Could you check a few things on this model? Use its own coordinates, in mm. Round coordinates to 2 decimals unless told otherwise and drop trailing zeros. Write each loop counter-clockwise with the first axis right and the second up, starting at its lowest first coordinate (ties: lowest second). Pieces come first, ordered by that corner, then holes. Notation, with made-up numbers: (-6.75, -28) -> (-2.75, -28) arc R7 ccw to (-2.75, -16) -> close; hole circle Ø10 at (-15, 76.25). An arc over 180 degrees is marked (long way). Answer as CSV lines item,"result". Start each with the question number.
Q1. Imagine slicing it at B-B on z = 57. Please give me the cut outline in (x, y), and give its area (3 significant figures).
Q2. If I drill on line 1 (X direction, y = -2, z = 0) (3 decimals); line 2 (Z direction, x = 64.5, y = -0.75); line 3 (Z direction, x = -53.5, y = -1.25), over which ranges is the centre line in solid material (lowest first)? Write a range as [from, to].
Q3. Imagine slicing it at C-C on x = -37.5. Please give me the cut outline in (y, z).
Q4. If we mould it in two halves opening along Y, with no side actions, what happens to faces 1 (the cylindrical face through (-21.993, -3.131, 69.635)), 2 (the flat face through (-3, 0, 0)), 3 (the flat face through (-3, -6.35, 0))? For each: pulls with the +Y half, pulls with the -Y half, needs draft (parallel to the pull), parting line crosses it, or undercut.
Q5. Will this pin go through, and if not, where does the flat tip stop? pin 1 Ø1.5 at (y, z) = (-3, 30) entering from +X.
from build123d import *

# Parameters (mm, degrees)
F1_DEPTH = 6.35
F2_DEPTH = 6.35


with BuildPart() as f1:
    # F0 (on Front) → F1 (new body)
    with BuildSketch(Plane.XZ):
        with BuildLine():
            ThreePointArc((46.19652, 60.349645), (43.160779, 59.896273), (40.267036, 60.919754))
            ThreePointArc((40.267036, 60.919754), (-22.87068, 69.351155), (-68.606756, 25.015267))
            ThreePointArc((-68.606756, 25.015267), (-70.323983, 22.471177), (-73.033881, 21.029748))
            ThreePointArc((-73.033881, 21.029748), (-77.712175, 16.161943), (-75.362586, 9.832537))
            ThreePointArc((-75.362586, 9.832537), (-73.452084, 7.430195), (-72.891573, 4.412399))
            ThreePointArc((-72.891573, 4.412399), (-48.624522, -54.482167), (12.639521, -71.922828))
            ThreePointArc((12.639521, -71.922828), (15.701382, -72.137945), (18.304645, -73.764071))
            ThreePointArc((18.304645, -73.764071), (24.859434, -75.38169), (29.166066, -70.182182))
            ThreePointArc((29.166066, -70.182182), (30.291304, -67.326468), (32.624537, -65.332153))
            ThreePointArc((32.624537, -65.332153), (71.495201, -14.868988), (55.967235, 46.90756))
            ThreePointArc((55.967235, 46.90756), (54.622602, 49.666768), (54.729237, 52.734323))
            ThreePointArc((54.729237, 52.734323), (52.852741, 59.219747), (46.19652, 60.349645))
        make_face()
    extrude(amount=F1_DEPTH)

    # F0 (on Front) → F2 (join)
    with BuildSketch(Plane.XZ):
        with BuildLine():
            ThreePointArc((46.19652, 60.349645), (43.160779, 59.896273), (40.267036, 60.919754))
            ThreePointArc((40.267036, 60.919754), (-22.87068, 69.351155), (-68.606756, 25.015267))
            ThreePointArc((-68.606756, 25.015267), (-70.323983, 22.471177), (-73.033881, 21.029748))
            ThreePointArc((-73.033881, 21.029748), (-77.712175, 16.161943), (-75.362586, 9.832537))
            ThreePointArc((-75.362586, 9.832537), (-73.452084, 7.430195), (-72.891573, 4.412399))
            ThreePointArc((-72.891573, 4.412399), (-48.624522, -54.482167), (12.639521, -71.922828))
            ThreePointArc((12.639521, -71.922828), (15.701382, -72.137945), (18.304645, -73.764071))
            ThreePointArc((18.304645, -73.764071), (24.859434, -75.38169), (29.166066, -70.182182))
            ThreePointArc((29.166066, -70.182182), (30.291304, -67.326468), (32.624537, -65.332153))
            ThreePointArc((32.624537, -65.332153), (71.495201, -14.868988), (55.967235, 46.90756))
            ThreePointArc((55.967235, 46.90756), (54.622602, 49.666768), (54.729237, 52.734323))
            ThreePointArc((54.729237, 52.734323), (52.852741, 59.219747), (46.19652, 60.349645))
        make_face()
    extrude(amount=F2_DEPTH)


solid = f1.part
Checks:
1,outline,"(-45.65, -6.35) -> (54.45, -6.35) -> (54.45, 0) -> (-45.65, 0) -> close"
1,area,"636 mm^2"
2,line 1,"[-73.025, 73.025]"
2,line 2,"[-34.24, 34.24]"
2,line 3,"[-49.7, 49.7]"
3,outline,"(-6.35, -62.66) -> (0, -62.66) -> (0, 62.66) -> (-6.35, 62.66) -> close"
4,face 1,"needs draft"
4,face 2,"pulls with the +Y half"
4,face 3,"pulls with the -Y half"
5,pin 1,"x = 66.91"
